The listing builds one solid part. Answer for the finished solid, in the listing's coordinates (mm). A direction names the side the tool comes from. Give positions to 0.01 mm unless a question says otherwise; leave off trailing zeros. Loops run counter-clockwise (first coordinate to the right, second up) from the corner with the lowest first, then second, coordinate; pieces in that order, holes last. Notation, with made-up numbers: (89.5, 78.25) - (132.5, 78.25) arc R14 cw to (132.5, 94.25) - close; hole circle Ø7 at (67, 77). An arc over 180 degrees is marked (long way). Answer as CSV lines item,"result". Start each with the question number.
1) Flat-ended cylindrical pins translate along their axes: pin 1 (2 mm diameter, centred on x = -6, y = 22, fed in from +Z); pin 2 (6 mm diameter, centred on x = -15.5, y = 9.5, fed in from +Z); pin 3 (6 mm diameter, centred on x = -16, y = 5, fed in from +Z). Find the tip coordinate at first contact, or state that the pin passes through.
2) A cutting plane is placed at C-C (y = 12). Determine the outline of the cut face in (x, z).
3) A cutting plane is placed at D-D (z = 3.25). Determine the outline of the cut face in (x, y).
4) For a pull along Y with two mould halves and no side action, classify faces 1 (the face through (-13.654, 20.021, 1.703)), 2 (the face through (-24, 12, 2)), 3 (the face through (-9, 24.5, 3)) as pulls with the +Y half, pulls with the -Y half, needs draft (parallel to the pull), parting line crosses it, or undercut.
5) For faces 4 (the face through (-4, 12, 11)), 5 (the face through (-1.972, 21.136, 9.215)), determine the directions among +Z, -Z, +X, -X, +Y, -Y from which every point of the face is accessible in a straight line to the end or side of a thin tool.
6) A cutting plane is placed at B-B (y = 5). Determine the outline of the cut face in (x, z), and give its area (3 significant figures).
7) A cutting plane is placed at A-A (z = 9). Determine the outline of the cut face in (x, y).
8) Find the intervals of material crossed by line 1 along Y through (x, z) = (-2.8, 9); line 2 along Y through (x, z) = (-16, 0.65); line 3 along X through (y, z) = (5, 1.05), in increasing order.
```python
from build123d import *

# Parameters (mm, degrees)
BOSS_EXTRUDE1_DEPTH                            = 24.5
CSK_FOR_M4_FLAT_HEAD_MACHINE_SCREW1_AT_2_COUNT = 2
CSK_FOR_M4_FLAT_HEAD_MACHINE_SCREW1_AT_2_PITCH = 14.5
TAP_DRILL_FOR_M4X0_7_TAP1_D                    = 3.3
FILLET1_R                                      = 3


with BuildPart() as part:
    # Sketch2 → Boss-Extrude1 (new body)
    with BuildSketch(Plane(origin=(0, 0, 0), x_dir=(1, 0, 0), z_dir=(0, 1, 0))):
        Polygon((0, 0), (-24, 0), (-24, -4), (-4, -4), (-4, -15), (0, -15), align=None)
    extrude(amount=BOSS_EXTRUDE1_DEPTH)

    # Sketch5 → CSK for M4 Flat Head Machine Screw1 (revolve, cut)
    with BuildSketch(Plane(origin=(-16, 5, 4), x_dir=(0, -1, 0), z_dir=(1, 0, 0))):
        Polygon((0, 0), (0, 4), (2.25, 4), (2.25, 2.45), (4.7, 0), align=None)
    csk_for_m4_flat_head_machine_screw1 = revolve(axis=Axis((-16, 5, 10.35), (0, 0, -1)), mode=Mode.SUBTRACT)

    # CSK for M4 Flat Head Machine Screw1 at 2: CSK for M4 Flat Head Machine Screw1 ×2
    with Locations(*[(0, i * CSK_FOR_M4_FLAT_HEAD_MACHINE_SCREW1_AT_2_PITCH, 0) for i in range(1, CSK_FOR_M4_FLAT_HEAD_MACHINE_SCREW1_AT_2_COUNT)]):
        add(csk_for_m4_flat_head_machine_screw1, mode=Mode.SUBTRACT)

    # Tap Drill for M4x0.7 Tap1 (through all)
    with Locations(Plane.ZY.offset(4)):
        with Locations((9, 5), (9, 19.5)):
            Hole(TAP_DRILL_FOR_M4X0_7_TAP1_D / 2)

    # Fillet1
    fillet1_edges = [part.edges().sort_by_distance(p)[0] for p in [
        (-4, 12.25, 4),
    ]]
    fillet(fillet1_edges, radius=FILLET1_R)


solid = part.part
```
Ans:
1,pin 1,"z = 4.76"
1,pin 2,"z = 4"
1,pin 3,"z = 2.3"
2,outline,"(-24, 0) - (0, 0) - (0, 15) - (-4, 15) - (-4, 7) arc R3 cw to (-7, 4) - (-24, 4) - close"
3,outline,"(-24, 0) - (0, 0) - (0, 24.5) - (-24, 24.5) - close; hole circle Ø7.9 at (-16, 5); hole circle Ø7.9 at (-16, 19.5)"
4,face 1,"undercut"
4,face 2,"needs draft"
4,face 3,"pulls with the +Y half"
5,face 4,"+Z, -X, +Y, -Y"
5,face 5,"+X, -X"
6,outline,"(-24, 0) - (-18.25, 0) - (-18.25, 1.55) - (-20.7, 4) - (-24, 4) - close; (-13.75, 0) - (0, 0) - (0, 7.35) - (-4, 7.35) - (-4, 7) arc R3 cw to (-7, 4) - (-11.3, 4) - (-13.75, 1.55) - close; (-4, 10.65) - (0, 10.65) - (0, 15) - (-4, 15) - close"
6,area,"105 mm2"
7,outline,"(-4, 0) - (0, 0) - (0, 3.35) - (-4, 3.35) - close; (-4, 6.65) - (0, 6.65) - (0, 17.85) - (-4, 17.85) - close; (-4, 21.15) - (0, 21.15) - (0, 24.5) - (-4, 24.5) - close"
8,line 1,"0 to 3.35, 6.65 to 17.85, 21.15 to 24.5"
8,line 2,"0 to 2.75, 7.25 to 17.25, 21.75 to 24.5"
8,line 3,"-24 to -18.25, -13.75 to 0"
